```python
from build123d import *

# Parameters (mm, degrees)
BOSS_EXTRUDE1_DEPTH   = 15
F_1_0MM_DOWEL_HOLE1_D = 10
BOSS_EXTRUDE2_DEPTH   = 15
ESCALA1_SCALE         = 0.2


with BuildPart() as part:
    # Sketch2 → Boss-Extrude1 (new body)
    with BuildSketch(Plane(origin=(0, 0, 0), x_dir=(1, 0, 0), z_dir=(0, 1, 0))):
        Polygon((-220, 30), (-220, -30), (-170, -90), (-50, -90), (-50, 90), (-170, 90), align=None)
    extrude(amount=BOSS_EXTRUDE1_DEPTH)

    # Ø1.0mm Dowel Hole1 (through all)
    with Locations(Plane(origin=(0, 15, 0), x_dir=(1, 0, 0), z_dir=(0, 1, 0))):
        with Locations((-204.389232105, 22.557395049), (-204.389232105, -22.557395049), (-112.996294866, 55), (-112.996294866, -55)):
            Hole(F_1_0MM_DOWEL_HOLE1_D / 2)

    # Sketch5 → Boss-Extrude2 (add)
    with BuildSketch(Plane(origin=(-50, 0, 0), x_dir=(0, 0, -1), z_dir=(1, 0, 0))):
        Polygon((-90, 15), (-55, 15), (-90, 45), align=None)
        Polygon((90, 45), (90, 15), (55, 15), align=None)
    extrude(amount=-BOSS_EXTRUDE2_DEPTH)


with BuildPart() as part_1:
    # Escala1: scaled about (-124.630859944, 8.148472024, 0)
    add(part.part.scale(ESCALA1_SCALE).moved(Location((-99.704687955, 6.518777619, 0))))


solid = part_1.part
```
Source: CAD feature listing. Evaluate the final solid. Frame: model axes, mm. A direction names the side the tool comes from. Coordinates: 2 decimals unless noted, no trailing zeros. Loops run counter-clockwise (first coordinate to the right, second up) from the corner with the lowest first, then second, coordinate; pieces in that order, holes last. Notation, with made-up numbers: M -26,39 L -5,39 A26 cw -5,65 Z; hole C -24.75,78 d5. An arc over 180 degrees is marked long. Use CSV: the item, a comma, the result in double quotes.
(1) Line query: line 1 (X direction, y = 7.75, z = 4.5); line 2 (Z direction, x = -122.5, y = 8.75); line 3 (Y direction, x = -111.5, z = 1). Output: solid intervals per line, ascending. Write a range as [from, to].
Answers follow:
line 1,"[-143.7, -141.58], [-139.58, -109.7]"
line 2,"[-18, -11.98], [-10.02, 10.02], [11.98, 18]"
line 3,"[6.52, 9.52]"
(2) Cut plane C-C on z = -13. Return loops of the section in (x, y), and give its area (3 significant figures).
Answers follow:
outline,"M -137.87,6.52 L -109.7,6.52 L -109.7,11.23 L -112.7,11.23 L -112.7,9.52 L -137.87,9.52 Z"
area,"89.6 mm²"
(3) Contact query for flat-ended pins moving along their axis: pin 1 (1.6 mm diameter, centred on x = -140.58, z = 4.51, fed in from -Y); pin 2 (5 mm diameter, centred on x = -119, z = 4, fed in from +Y); pin 3 (1.8 mm diameter, centred on y = 11.5, z = 16, fed in from -X). Output: stop coordinate, or through.
Answers follow:
pin 1,"through"
pin 2,"y = 9.52"
pin 3,"x = -112.7"
(4) Draft query along X for faces 4 (the face through (-127, 9.519, 0)), 5 (the face through (-109.705, 9, 0)), 6 (the face through (-141.536, 7.998, 4.211)). Return one class per face: pulls with the +X half, pulls with the -X half, needs draft (parallel to the pull), parting line crosses it, or undercut.
Answers follow:
face 4,"needs draft"
face 5,"pulls with the +X half"
face 6,"undercut"
(5) Reachability of faces 1 (the face through (-111.184, 12.477, 14.451)), 2 (the face through (-112.705, 11, 16)), 3 (the face through (-138.77, 8, 11.92)) from +Z, -Z, +X, -X, +Y, -Y: full face, straight path, thin tool, end or side. Return the list, or none.
Answers follow:
face 1,"+X, -X, +Y"
face 2,"+Z, -Z, -X, +Y"
face 3,"+Z, -X, +Y, -Y"
(6) Cut plane D-D on x = -131. Return loops of the section in (y, z).
Answers follow:
outline,"M 6.52,-18 L 9.52,-18 L 9.52,18 L 6.52,18 Z"
(7) Cut plane B-B on y = 8.75. Return loops of the section in (x, z).
Answers follow:
outline,"M -143.7,-6 L -133.7,-18 L -109.7,-18 L -109.7,18 L -133.7,18 L -143.7,6 Z; hole C -140.58,-4.51 d2; hole C -140.58,4.51 d2; hole C -122.3,-11 d2; hole C -122.3,11 d2"
(8) Cut plane A-A on y = 15. Return loops of the section in (x, z).
Answers follow:
outline,"M -112.7,-18 L -109.7,-18 L -109.7,-17.39 L -112.7,-17.39 Z; M -112.7,17.39 L -109.7,17.39 L -109.7,18 L -112.7,18 Z"
